Geometry check sheet. Reference: the model listing, model coordinates, mm. A direction names the side the tool comes from. Give positions to 0.01 mm unless a question says otherwise; leave off trailing zeros. Order: outer loops, then holes, each group sorted by start corner. A loop starts at its lowest first (then second) coordinate and runs counter-clockwise, first axis right, second up. Notation, with made-up numbers: M 68.5,59 L 95.5,59 A34 cw 95.5,90 Z; hole C -11.5,41.25 d2. An arc over 180 degrees is marked long. Answer as CSV lines item,"result". Start each with the question number.
```python
from build123d import *

# Parameters (mm, degrees)
CUT_EXTRUDE3_REACH = 8
SKETCH4_R          = 1.25
SKETCH2_R          = 12
CUT_EXTRUDE4_DEPTH = 1
CUT_EXTRUDE5_REACH = 7
SKETCH5_R          = 7.2


with BuildPart() as part:
    # Sketch1 → Revolve1 (revolve)
    with BuildSketch(Plane.XY):
        Polygon((0, 0), (0, 17), (2, 17), (2, 12), (6, 12), (6, 10), (2, 9), (2, 0), align=None)
    revolve(axis=Axis((0, 0, 0), (1, 0, 0)))

    # Sketch4 → Cut-Extrude3 (cut, up to next)
    with BuildSketch(Plane.ZY, mode=Mode.PRIVATE) as cut_extrude3_sk1:
        with Locations((0, 14)):
            Circle(SKETCH4_R)
    cut_extrude3_tool1 = extrude(cut_extrude3_sk1.sketch, amount=-CUT_EXTRUDE3_REACH, mode=Mode.PRIVATE) & part.part
    add(cut_extrude3_tool1.solids().sort_by_distance((0, 14, 0))[0], mode=Mode.SUBTRACT)
    # Sketch4 → Cut-Extrude3 (cut, up to next)
    with BuildSketch(Plane.ZY, mode=Mode.PRIVATE) as cut_extrude3_sk2:
        with Locations((14, 0)):
            Circle(SKETCH4_R)
    cut_extrude3_tool2 = extrude(cut_extrude3_sk2.sketch, amount=-CUT_EXTRUDE3_REACH, mode=Mode.PRIVATE) & part.part
    add(cut_extrude3_tool2.solids().sort_by_distance((0, 0, 14))[0], mode=Mode.SUBTRACT)
    # Sketch4 → Cut-Extrude3 (cut, up to next)
    with BuildSketch(Plane.ZY, mode=Mode.PRIVATE) as cut_extrude3_sk3:
        with Locations((0, -14)):
            Circle(SKETCH4_R)
    cut_extrude3_tool3 = extrude(cut_extrude3_sk3.sketch, amount=-CUT_EXTRUDE3_REACH, mode=Mode.PRIVATE) & part.part
    add(cut_extrude3_tool3.solids().sort_by_distance((0, -14, 0))[0], mode=Mode.SUBTRACT)
    # Sketch4 → Cut-Extrude3 (cut, up to next)
    with BuildSketch(Plane.ZY, mode=Mode.PRIVATE) as cut_extrude3_sk4:
        with Locations((-14, 0)):
            Circle(SKETCH4_R)
    cut_extrude3_tool4 = extrude(cut_extrude3_sk4.sketch, amount=-CUT_EXTRUDE3_REACH, mode=Mode.PRIVATE) & part.part
    add(cut_extrude3_tool4.solids().sort_by_distance((0, 0, -14))[0], mode=Mode.SUBTRACT)

    # Sketch2 → Cut-Extrude4 (cut)
    with BuildSketch(Plane.ZY):
        Circle(SKETCH2_R)
    extrude(amount=-CUT_EXTRUDE4_DEPTH, mode=Mode.SUBTRACT)

    # Sketch5 → Cut-Extrude5 (cut, up to next)
    with BuildSketch(Plane.ZY.offset(-1), mode=Mode.PRIVATE) as cut_extrude5_sk1:
        Circle(SKETCH5_R)
    cut_extrude5_tool1 = extrude(cut_extrude5_sk1.sketch, amount=-CUT_EXTRUDE5_REACH, mode=Mode.PRIVATE) & part.part
    add(cut_extrude5_tool1.solids().sort_by_distance((1, 0, 0))[0], mode=Mode.SUBTRACT)


solid = part.part
```
Item 1: Depth check by flat-ended pin: pin 1 Ø5.5 at (y, z) = (3.5, 0) entering from +X; pin 2 Ø2 at (x, z) = (1.5, 8) entering from -Y; pin 3 Ø3 at (x, z) = (4.5, 7) entering from -Y; pin 4 Ø3 at (y, z) = (0, 14) entering from +X. Enter the tip coordinate at first touch or a pass-through.
Item 2: Scan lines: line 1 along X through (y, z) = (2, -16); line 2 along Z through (x, y) = (1.15, -13); line 3 along Y through (x, z) = (2.85, -1.5). Record each from-to range of solid material in increasing order.
Item 3: Access from +Z, -Z, +X, -X, +Y, -Y to the whole of each face (thin tool, end or side, straight path). Record for faces 1 (the face through (4.03, -11.99, 0.53)), 2 (the face through (0.49, 0.53, -11.99)), 3 (the face through (0.99, -12.76, -0.16)).
Item 4: Section check C-C on z = 14. Record the boundary of the cut face in (x, y), then the cut area to 3 significant figures.
Item 5: Section check A-A on y = 0. Record the boundary of the cut face in (x, z).
Item 6: Draft check along Y on faces 4 (the face through (2.194, -1.962, -8.833)), 5 (the face through (0, 4, 12)), 6 (the face through (1.014, 9.139, 14.334)). Enter one of: pulls with the +Y half, pulls with the -Y half, needs draft (parallel to the pull), parting line crosses it, or undercut.
Numbers:
1,pin 1,"through"
1,pin 2,"y = -15.49"
1,pin 3,"y = -10.67"
1,pin 4,"x = 2"
2,line 1,"0 to 2"
2,line 2,"-10.95 to -0.75, 0.75 to 10.95"
2,line 3,"-11.91 to -9.09, 9.09 to 11.91"
3,face 1,"+X"
3,face 2,"-X"
3,face 3,"+X, -X"
4,outline,"M 0,-9.64 L 2,-9.64 L 2,-1.25 L 0,-1.25 Z; M 0,1.25 L 2,1.25 L 2,9.64 L 0,9.64 Z"
4,area,"33.6 mm2"
5,outline,"M 0,-17 L 2,-17 L 2,-15.25 L 0,-15.25 Z; M 0,-12.75 L 2,-12.75 L 2,-12 L 6,-12 L 6,-10 L 2,-9 L 2,-7.2 L 1,-7.2 L 1,-12 L 0,-12 Z; M 0,12 L 1,12 L 1,7.2 L 2,7.2 L 2,9 L 6,10 L 6,12 L 2,12 L 2,12.75 L 0,12.75 Z; M 0,15.25 L 2,15.25 L 2,17 L 0,17 Z"
6,face 4,"undercut"
6,face 5,"needs draft"
6,face 6,"parting line crosses it"
